Work out the finished part from the listing and answer in its coordinate system (mm). A direction names the side the tool comes from. Round coordinates to 2 decimals unless told otherwise and drop trailing zeros. Loops run counter-clockwise (first coordinate to the right, second up) from the corner with the lowest first, then second, coordinate; pieces in that order, holes last.
Autodesk Inventor part; units mm, degrees
ref_plane "YZ Plane" through (0, 0, 0) normal (1, 0, 0) x (0, 1, 0)
ref_plane "XZ Plane" through (0, 0, 0) normal (0, 1, 0) x (-1, 0, 0)
ref_plane "XY Plane" through (0, 0, 0) normal (0, 0, 1) x (1, 0, 0)
sketch "Sketch1" plane through (0, 0, 0) normal (0, 0, 1) x (1, 0, 0)
  circle A0 centre (0, 0) radius 7
  circle A1 centre (0, 0) radius 16
  dimension "d0" = 32
  dimension "d1" = 14
extrude "Extrusion1" add sketch "Sketch1" along normal blind 1
sketch "Sketch2" plane through (0, 0, 1) normal (0, 0, 1) x (1, 0, 0)
  circle A0 centre (9, 0) radius 2.6
  point P0 (0, 0)
  dimension "d4" = 9
  dimension "d5" = 5.2
extrude "Extrusion2" cut sketch "Sketch2" against normal blind 1
pattern_circular "Circular Pattern1" count 3 over 360 about axis through (0, 0, 0) along (0, 0, 1) of "Extrusion2"
sketch "Sketch4" plane through (0, 0, 1) normal (0, 0, 1) x (1, 0, 0)
  arc A0 (-2.1614, 6.6579) -> (-4.6852, 5.2008) centre (-4.5, 7.7942) ccw
  circle A1 centre (-4.5, 7.7942) radius 5
  arc A2 (-4.6852, -5.2008) -> (-2.1614, -6.6579) centre (-4.5, -7.7942) ccw
  circle A3 centre (-4.5, -7.7942) radius 5
  point P0 (0, 0)
  dimension "d12" = 10
extrude "Extrusion3" cut sketch "Sketch4" against normal through all
sketch "Sketch5" plane through (0, 0, 1) normal (0, 0, 1) x (1, 0, 0)
  arc A0 (6.8467, -1.4571) -> (6.8467, 1.4571) centre (9, 0) ccw
  circle A1 centre (9, 0) radius 4
  circle A2 centre (9, 0) radius 2.6
  point P0 (0, 0)
  point P1 (6.8467, 1.4571)
  dimension "d16" = 8
extrude "Extrusion4" add sketch "Sketch5" against normal up to surface (1 mm away)
fillet "Fillet3" radius 2 6 edges at (0.4343, 6.9865, 0.5) (-6.2677, 3.1171, 0.5) (-6.2677, -3.1171, 0.5) (0.4343, -6.9865, 0.5) (6.3333, -2.9814, 0.5) (6.3333, 2.9814, 0.5)
properties part number "ring-pre-anode" material "Stainless Steel"
Item 1: For faces 4 (the face through (3.88, -5.826, 0.493)), 5 (the face through (7, -3, 1)), determine the directions among +Z, -Z, +X, -X, +Y, -Y from which every point of the face is accessible in a straight line to the end or side of a thin tool.
Item 2: Section B-B, the plane x = 9 is taken. Give the vertices of the cut face in (y, z), plus the area to 3 significant figures.
Item 3: Section D-D, the plane z = 0.8 is taken. State how many separate pieces and enclosed holes the cut face has, plus the area to 3 significant figures.
Item 4: Determine the mould class of faces 1 (the face through (7, -3, 0)), 2 (the face through (5, 0, 0.5)), 3 (the face through (-3.47, 15.62, 0.49)) for opening direction X: pulls with the +X half, pulls with the -X half, needs draft (parallel to the pull), parting line crosses it, or undercut.
Item 5: Straight lines are drawn through the part: line 1 (X direction, y = 3, z = 0.85); line 2 (X direction, y = 5, z = 0.45); line 3 (Y direction, x = 1, z = 0.35). For each, find the intervals that lie inside material, in ascending order.
Item 6: This flat-tipped pin is pushed along its axis until it touches: P1, Ø8, axis at x = 11.5, y = -3.5, coming from the -Z side. Where does it stop, or does it pass through?
Item 7: Section A-A, the plane y = 0 is taken. Give the vertices of the cut face in (x, z), plus the area to 3 significant figures.
Item 8: Section C-C, the plane y = -10 is taken. Give the vertices of the cut face in (x, z).
Answer below:
1. face 4: +Z, -Z
1. face 5: +Z, +X, -X, +Y, -Y
2. outline: (-13.23, 0) - (-2.6, 0) - (-2.6, 1) - (-13.23, 1) - close; (2.6, 0) - (13.23, 0) - (13.23, 1) - (2.6, 1) - close
2. area: 21.3 mm2
3. separate pieces: 1
3. enclosed holes: 2
3. area: 511 mm2
4. face 1: needs draft
4. face 2: undercut
4. face 3: parting line crosses it
5. line 1: x = -15.72 to -6.89, 5.88 to 15.72
5. line 2: x = -15.2 to -8.65, 4.9 to 15.2
5. line 3: y = -15.97 to -7.28, 7.28 to 15.97
6. P1: stops at z = 0
7. outline: (-16, 0) - (-7, 0) - (-7, 1) - (-16, 1) - close; (5, 0) - (6.4, 0) - (6.4, 1) - (5, 1) - close; (11.6, 0) - (16, 0) - (16, 1) - (11.6, 1) - close
7. area: 14.8 mm2
8. outline: (-12.49, 0) - (-8.99, 0) - (-8.99, 1) - (-12.49, 1) - close; (-0.01, 0) - (12.49, 0) - (12.49, 1) - (-0.01, 1) - close
